Geometry: final body of the model. Coordinates: model frame, mm. A direction names the side the tool comes from. Give positions to 0.01 mm unless a question says otherwise; leave off trailing zeros. Write each loop counter-clockwise with the first axis right and the second up, starting at its lowest first coordinate (ties: lowest second). Pieces come first, ordered by that corner, then holes.
Q1. Mould query, pull axis Z, two halves, no side actions, for faces 1 (the flat face through (39.742, 2, 36)), 2 (the cylindrical face through (20.157, -8.146, 65.236)), 3 (the flat face through (20, 1, -3.148)). Classes: +Z half, -Z half, draft (parallel to the pull), parting line (faces both ways), or undercut.
Q2. Line query: line 1 (X direction, y = 2, z = 32.5); line 2 (Y direction, x = 30.5, z = 45.5); line 3 (Z direction, x = 27.5, y = -4). Output: solid intervals per line, ascending.
Q3. Section A-A (z = 23). Return the cut outline in (x, y).
Q4. Pin query (flat end, axial travel): pin 1 Ø0.5 at (y, z) = (2, 37) entering from -X; pin 2 Ø0.9 at (x, y) = (28.5, 2) entering from -Z; pin 3 Ø5 at (y, z) = (-7, 41.5) entering from +X. Return the tip coordinate at first contact, or that it passes through.
Q5. Section B-B (x = 17). Return the cut outline in (y, z).
Q6. Section C-C (y = -1.5). Return the cut outline in (x, z).
Q7. Reachability of faces 4 (the flat face through (6, 2, 71.613)), 5 (the flat face through (28.323, 1, 70)), 6 (the flat face through (-1.197, 2, 67)), 7 (the flat face through (20, 1.453, 35)) from +Z, -Z, +X, -X, +Y, -Y: full face, straight path, thin tool, end or side. Return the list, or none.
Q8. Section D-D (x = 6.5). Return the cut outline in (y, z).
from build123d import *

# Parameters (mm, degrees)
PCB_DIMENSIONS_W    = 47.716732244
PCB_DIMENSIONS_H    = 77.636732244
BOSS_EXTRUDE3_DEPTH = 1.5
SKETCH5_W           = 43.474091557
SKETCH5_H           = 73.394091557
SKETCH5_W_2         = 39.23145087
SKETCH5_H_2         = 69.15145087
BOSS_EXTRUDE4_DEPTH = 1.8
FILLET1_R           = 1
SKETCH6_W           = 12
SKETCH6_H           = 31.966906412
SKETCH6_H_2         = 32.033093588
BOSS_EXTRUDE5_DEPTH = 10
SKETCH7_W           = 48
SKETCH7_H           = 6
CUT_EXTRUDE1_DEPTH  = 24
FILLET2_R           = 6
FILLET3_R           = 1
SCALE1_SCALE        = 0.99
CUT_EXTRUDE2_DEPTH  = 10
SKETCH9_W           = 7
SKETCH9_H           = 8.5
CUT_EXTRUDE3_DEPTH  = 10


with BuildPart() as part:
    # PCB Dimensions → Boss-Extrude3 (new body)
    with BuildSketch(Plane(origin=(0, 0, 0), x_dir=(1, 0, 0), z_dir=(0, 1, 0))):
        with Locations((20.322832216, -35.282832216)):
            Rectangle(PCB_DIMENSIONS_W, PCB_DIMENSIONS_H)
    extrude(amount=BOSS_EXTRUDE3_DEPTH)

    # Sketch5 → Boss-Extrude4 (add)
    with BuildSketch(Plane(origin=(0, 1.5, 0), x_dir=(1, 0, 0), z_dir=(0, 1, 0))):
        with Locations((20.322832217, -35.282832217)):
            Rectangle(SKETCH5_W, SKETCH5_H)
        with Locations((20.322832216, -35.282832216)):
            Rectangle(SKETCH5_W_2, SKETCH5_H_2, mode=Mode.SUBTRACT)
    extrude(amount=BOSS_EXTRUDE4_DEPTH)

    # Fillet1
    fillet1_edges = [part.edges().sort_by_distance(p)[0] for p in [
        (-1.414213562, 2.4, -1.414213562),
        (-1.414213562, 2.4, 71.979877995),
        (42.059877995, 2.4, 71.979877995),
        (42.059877995, 2.4, -1.414213562),
        (0.707106781, 2.4, 0.707106781),
        (0.707106781, 2.4, 69.858557651),
        (39.938557651, 2.4, 69.858557651),
        (39.938557651, 2.4, 0.707106781),
    ]]
    fillet(fillet1_edges, radius=FILLET1_R)

    # Sketch6 → Boss-Extrude5 (add)
    with BuildSketch(Plane.XZ):
        with Locations((14.322832216, 51.266285422)):
            Rectangle(SKETCH6_W, SKETCH6_H)
        with Locations((26.322832216, 51.266285422)):
            Rectangle(SKETCH6_W, SKETCH6_H)
        with Locations((14.322832216, 19.266285422)):
            Rectangle(SKETCH6_W, SKETCH6_H_2)
        with Locations((26.322832216, 19.266285422)):
            Rectangle(SKETCH6_W, SKETCH6_H_2)
    extrude(amount=BOSS_EXTRUDE5_DEPTH)

    # Sketch7 → Cut-Extrude1 (cut)
    with BuildSketch(Plane(origin=(32.322832216, 0, 0), x_dir=(0, 0, -1), z_dir=(1, 0, 0))):
        with Locations((-35.249738628, -3)):
            Rectangle(SKETCH7_W, SKETCH7_H)
    extrude(amount=-CUT_EXTRUDE1_DEPTH, mode=Mode.SUBTRACT)

    # Fillet2
    fillet2_edges = [part.edges().sort_by_distance(p)[0] for p in [
        (20.322832216, -10, 67.249738628),
        (20.322832216, -10, 3.249738628),
    ]]
    fillet(fillet2_edges, radius=FILLET2_R)

    # Fillet3
    fillet3_edges = [part.edges().sort_by_distance(p)[0] for p in [
        (20.322832216, -6, 59.249738628),
        (20.322832216, -6, 11.249738628),
    ]]
    fillet(fillet3_edges, radius=FILLET3_R)


with BuildPart() as part_1:
    # Scale1: scaled about (20.322832216, -3.218350849, 35.264379677)
    add(part.part.scale(SCALE1_SCALE).moved(Location((0.203228322, -0.032183508, 0.352643797))))

    # Sketch8 → Cut-Extrude2 (cut)
    with BuildSketch(Plane.XZ.offset(0.032183508)):
        Polygon((20.322832216, 73.712830152), (12.322832216, 73.712830152), (12.322832216, 66.929885038), (28.322832216, 66.929885038), (28.322832216, 73.712830152), align=None)
    extrude(amount=-CUT_EXTRUDE2_DEPTH, mode=Mode.SUBTRACT)

    # Sketch9 → Cut-Extrude3 (cut)
    with BuildSketch(Plane.XZ.offset(0.032183508)):
        with Locations((0.203049755, 59.862830152)):
            Rectangle(SKETCH9_W, SKETCH9_H)
    extrude(amount=-CUT_EXTRUDE3_DEPTH, mode=Mode.SUBTRACT)


solid = part_1.part
Computed:
1. face 1: undercut
1. face 2: +Z half
1. face 3: -Z half
2. line 1: x = -1.2 to 0.9, 39.74 to 41.84
2. line 2: y = -9.93 to -5.97, -0.03 to 1.45
2. line 3: z = 3.57 to 11.49, 59.01 to 66.93
3. outline: (-3.3, -0.03) - (43.94, -0.03) - (43.94, 1.45) - (41.84, 1.45) - (41.84, 3.23) - (39.74, 3.23) - (39.74, 1.45) - (0.9, 1.45) - (0.9, 3.23) - (-1.2, 3.23) - (-1.2, 1.45) - (-3.3, 1.45) - close; (8.44, -9.93) - (32.2, -9.93) - (32.2, -5.97) - (8.44, -5.97) - close
4. pin 1: stops at x = -1.2
4. pin 2: stops at z = -1.05
4. pin 3: stops at x = 32.2
5. outline: (-9.93, 9.51) arc R5.94 ccw to (-3.99, 3.57) - (-0.03, 3.57) - (-0.03, -3.15) - (1.45, -3.15) - (1.45, -1.05) - (3.23, -1.05) - (3.23, 1.05) - (1.45, 1.05) - (1.45, 66.93) - (-3.99, 66.93) arc R5.94 ccw to (-9.93, 60.99) - close; hole (-5.97, 12.48) arc R0.99 ccw to (-4.98, 11.49) - (-0.03, 11.49) - (-0.03, 59.01) - (-4.98, 59.01) arc R0.99 ccw to (-5.97, 58.02) - close
6. outline: (8.44, 3.57) - (32.2, 3.57) - (32.2, 11.49) - (8.44, 11.49) - close; (8.44, 59.01) - (32.2, 59.01) - (32.2, 66.93) - (8.44, 66.93) - close
7. face 4: +Z, +X, -X, +Y
7. face 5: +Z, +Y, -Y
7. face 6: +Z, -Z, -X, +Y
7. face 7: +Y
8. outline: (-0.03, -3.15) - (1.45, -3.15) - (1.45, -1.05) - (3.23, -1.05) - (3.23, 1.05) - (1.45, 1.05) - (1.45, 69.51) - (3.23, 69.51) - (3.23, 71.61) - (1.45, 71.61) - (1.45, 73.71) - (-0.03, 73.71) - close
